Check sheet for the modelled part. Datum: model origin and axes. Units: mm. Face numbers are marked on the shaded views. A direction names the side the tool comes from. Give positions to 0.01 mm unless a question says otherwise; leave off trailing zeros. Write each loop counter-clockwise with the first axis right and the second up, starting at its lowest first coordinate (ties: lowest second). Pieces come first, ordered by that corner, then holes. Notation, with made-up numbers: M 49.25,61.5 L 87.25,61.5 A17 ccw 87.25,76.5 Z; hole C -28,-8 d3. An arc over 180 degrees is marked long. Write item = value, one per line. Start each with the question number.
1) Cross-section at B-B, the plane z = 5. Record the cut outline in (x, y).
2) Access from +Z, -Z, +X, -X, +Y, -Y to the whole of each face (thin tool, end or side, straight path). Record for the marked faces 4, 5 and 6.
3) Cross-section at A-A, the plane x = 0. Record the cut outline in (y, z), plus the area to 3 significant figures.
4) Cross-section at D-D, the plane x = -10. Record the cut outline in (y, z), plus the area to 3 significant figures.
5) Go/stop test with flat-tipped pins: pin 1 (5 mm diameter, centred on y = 22, z = 4, fed in from +X); pin 2 (4 mm diameter, centred on x = -18, z = 7, fed in from +Y); pin 3 (4 mm diameter, centred on x = 0, y = 32, fed in from +Z); pin 4 (1.5 mm diameter, centred on x = -0.5, z = 1.5, fed in from +Y). Record where each tip stops, or that it passes through.
6) Mould release check, pull along Y, two halves, no side actions. Record for the marked faces 1, 2 and 3: released by +Y, released by -Y, zero draft, split by the parting line, or undercut.
7) Cross-section at C-C, the plane y = 0. Record the cut outline in (x, z).
8) Scan lines: line 1 along X through (y, z) = (0, 4.5); line 2 along Y through (x, z) = (0, 3.75); line 3 along Z through (x, y) = (15, -2). Record each from-to range of solid material in increasing order. Write a range as [from, to].
```python
from build123d import *

# Parameters (mm, degrees)
SKETCH_1_R          = 2.25
EXTRUDE_1_DEPTH     = 10
CUT_EXTRUDE_1_DEPTH = 3


with BuildPart() as part:
    # 草图1 → 凸台-拉伸1 (new body)
    with BuildSketch(Plane.XY):
        with BuildLine():
            Line((-20, 12), (-20, -8))
            Line((-20, -8), (20, -8))
            Line((20, -8), (20, 12))
            Line((20, 12), (16.5, 12))
            ThreePointArc((16.5, 12), (13.671572875, 13.171572875), (12.5, 16))
            Line((12.5, 16), (12.5, 32))
            ThreePointArc((12.5, 32), (0, 44.5), (-12.5, 32))
            Line((-12.5, 32), (-12.5, 16))
            ThreePointArc((-12.5, 16), (-13.671572875, 13.171572875), (-16.5, 12))
            Line((-16.5, 12), (-20, 12))
        make_face()
        with Locations((-11.5, 0)):
            Circle(SKETCH_1_R, mode=Mode.SUBTRACT)
        with Locations((11.5, 0)):
            Circle(SKETCH_1_R, mode=Mode.SUBTRACT)
        with Locations((0, 32)):
            Circle(SKETCH_1_R, mode=Mode.SUBTRACT)
    extrude(amount=EXTRUDE_1_DEPTH)

    # 草图2 → 切除-拉伸1 (cut)
    with BuildSketch(Plane(origin=(0, 0, 0), x_dir=(-1, 0, 0), z_dir=(0, 0, -1))):
        Polygon((-11.5, -4.330127019), (-7.75, -2.165063509), (-7.75, 2.165063509), (-11.5, 4.330127019), (-15.25, 2.165063509), (-15.25, -2.165063509), align=None)
        Polygon((11.5, -4.330127019), (15.25, -2.165063509), (15.25, 2.165063509), (11.5, 4.330127019), (7.75, 2.165063509), (7.75, -2.165063509), align=None)
    extrude(amount=-CUT_EXTRUDE_1_DEPTH, mode=Mode.SUBTRACT)


solid = part.part
```
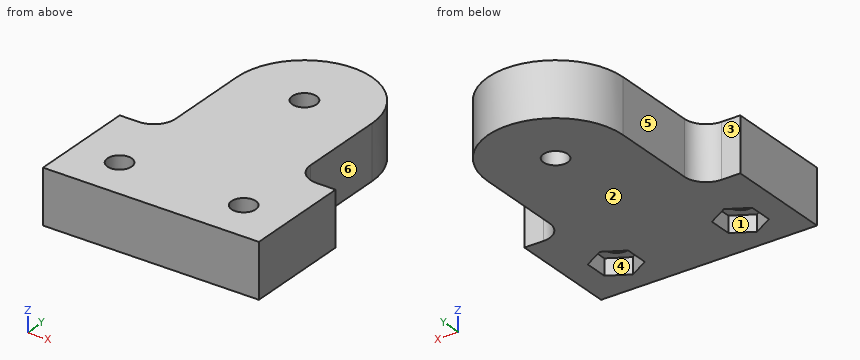
Reply:
q1.outline = M -20,-8 L 20,-8 L 20,12 L 16.5,12 A4 cw 12.5,16 L 12.5,32 A12.5 ccw -12.5,32 L -12.5,16 A4 cw -16.5,12 L -20,12 Z; hole C -11.5,0 d4.5; hole C 0,32 d4.5; hole C 11.5,0 d4.5
q2.face_4 = -Z
q2.face_5 = +Z, -Z, -X, +Y
q2.face_6 = +Z, -Z, +X, +Y
q3.outline = M -8,0 L 29.75,0 L 29.75,10 L -8,10 Z; M 34.25,0 L 44.5,0 L 44.5,10 L 34.25,10 Z
q3.area = 480 mm2
q4.outline = M -8,0 L -3.46,0 L -3.46,3 L -1.68,3 L -1.68,10 L -8,10 Z; M 1.68,3 L 3.46,3 L 3.46,0 L 39.5,0 L 39.5,10 L 1.68,10 Z
q4.area = 431 mm2
q5.pin_1 = 12.5
q5.pin_2 = 12.03
q5.pin_3 = through
q5.pin_4 = 44.5
q6.face_1 = undercut
q6.face_2 = zero draft
q6.face_3 = released by +Y
q7.outline = M -20,0 L -15.25,0 L -15.25,3 L -13.75,3 L -13.75,10 L -20,10 Z; M -9.25,3 L -7.75,3 L -7.75,0 L 7.75,0 L 7.75,3 L 9.25,3 L 9.25,10 L -9.25,10 Z; M 13.75,3 L 15.25,3 L 15.25,0 L 20,0 L 20,10 L 13.75,10 Z
q8.line_1 = [-20, -13.75], [-9.25, 9.25], [13.75, 20]
q8.line_2 = [-8, 29.75], [34.25, 44.5]
q8.line_3 = [3, 10]
